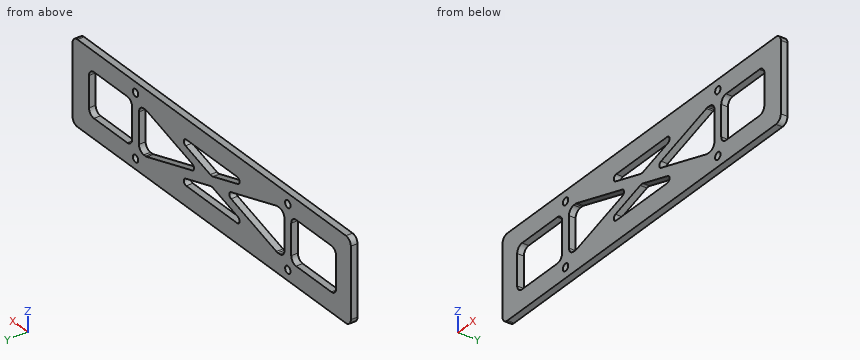
```python
from build123d import *

# Parameters (mm, degrees)
SKETCH1_W           = 145.0086
SKETCH1_H           = 32.004
SKETCH1_R           = 1.399999994
SKETCH1_R_2         = 1.399999995
SKETCH1_W_2         = 22.457386235
SKETCH1_H_2         = 16.9672
SKETCH1_W_3         = 23.43040653
BOSS_EXTRUDE1_DEPTH = 2.54
FILLET1_R           = 2.54
FILLET2_R           = 1.27


with BuildPart() as part:
    # Sketch1 → Boss-Extrude1 (new body)
    with BuildSketch(Plane(origin=(0, 0, 0), x_dir=(1, 0, 0), z_dir=(0, 1, 0))):
        with Locations((6.69779506, 14.755388179)):
            Rectangle(SKETCH1_W, SKETCH1_H)
        with Locations(Location((-32.97809841, 26.794988179, 0), (0, 0, 270))):
            Circle(SKETCH1_R, mode=Mode.SUBTRACT)
        with Locations(Location((46.373688528, 26.794988179, 0), (0, 0, 90))):
            Circle(SKETCH1_R_2, mode=Mode.SUBTRACT)
        with Locations(Location((46.373688528, 2.715788179, 0), (0, 0, 270))):
            Circle(SKETCH1_R_2, mode=Mode.SUBTRACT)
        with Locations(Location((-32.97809841, 2.715788179, 0), (0, 0, 90))):
            Circle(SKETCH1_R, mode=Mode.SUBTRACT)
        Polygon((-31.20009841, 23.238988179), (-27.382615546, 23.238988179), (0.574659599, 14.755388179), (-27.382615546, 6.271788179), (-31.20009841, 6.271788179), align=None, mode=Mode.SUBTRACT)
        with Locations((59.380381646, 14.755388179)):
            Rectangle(SKETCH1_W_2, SKETCH1_H_2, mode=Mode.SUBTRACT)
        with Locations((-46.471301675, 14.755388179)):
            Rectangle(SKETCH1_W_3, SKETCH1_H_2, mode=Mode.SUBTRACT)
        Polygon((40.778205663, 23.238988179), (12.820930519, 14.755388179), (40.778205663, 6.271788179), (44.595688528, 6.271788179), (44.595688528, 23.238988179), align=None, mode=Mode.SUBTRACT)
        Polygon((-15.136344626, 23.238988179), (6.697795059, 16.613445937), (28.531934744, 23.238988179), align=None, mode=Mode.SUBTRACT)
        Polygon((6.697795059, 12.897330421), (-15.136344626, 6.271788179), (28.531934744, 6.271788179), align=None, mode=Mode.SUBTRACT)
    extrude(amount=BOSS_EXTRUDE1_DEPTH)

    # Fillet1
    fillet1_edges = [part.edges().sort_by_distance(p)[0] for p in [
        (70.609074763, 1.27, -6.271788179),
        (70.609074763, 1.27, -23.238988179),
        (48.151688528, 1.27, -23.238988179),
        (48.151688528, 1.27, -6.271788179),
        (-58.18650494, 1.27, -23.238988179),
        (-58.18650494, 1.27, -6.271788179),
        (-34.75609841, 1.27, -6.271788179),
        (-34.75609841, 1.27, -23.238988179),
        (6.697795059, 1.27, -16.613445937),
        (6.697795059, 1.27, -12.897330421),
        (79.20209506, 1.27, 1.246611821),
        (-65.80650494, 1.27, 1.246611821),
        (-65.80650494, 1.27, -30.757388179),
        (79.20209506, 1.27, -30.757388179),
        (44.595688528, 1.27, -23.238988179),
        (40.778205663, 1.27, -23.238988179),
        (40.778205663, 1.27, -6.271788179),
        (44.595688528, 1.27, -6.271788179),
        (-31.20009841, 1.27, -23.238988179),
        (-31.20009841, 1.27, -6.271788179),
        (-27.382615546, 1.27, -6.271788179),
        (-27.382615546, 1.27, -23.238988179),
    ]]
    fillet(fillet1_edges, radius=FILLET1_R)

    # Fillet2
    fillet2_edges = [part.edges().sort_by_distance(p)[0] for p in [
        (28.531934744, 1.27, -23.238988179),
        (-15.136344626, 1.27, -23.238988179),
        (-15.136344626, 1.27, -6.271788179),
        (28.531934744, 1.27, -6.271788179),
        (12.820930519, 1.27, -14.755388179),
        (0.574659599, 1.27, -14.755388179),
    ]]
    fillet(fillet2_edges, radius=FILLET2_R)


solid = part.part
```
Geometry: final body of the model. Coordinates: model frame, mm. Coordinates: 2 decimals unless noted, no trailing zeros. Order: outer loops, then holes, each group sorted by start corner. A loop starts at its lowest first (then second) coordinate and runs counter-clockwise, first axis right, second up.
Item 1: Section query B-B (x = 4). Output: boundary loops of the cut face in (y, z), then the cut area to 3 significant figures.
Answer:
outline: (0, -30.76) - (2.54, -30.76) - (2.54, -23.24) - (0, -23.24) - close; (0, -17.43) - (2.54, -17.43) - (2.54, -12.08) - (0, -12.08) - close; (0, -6.27) - (2.54, -6.27) - (2.54, 1.25) - (0, 1.25) - close
area: 51.8 mm2
Item 2: Material intervals for line 1 along X through (y, z) = (2.25, -27); line 2 along Z through (x, y) = (-55, 0.9); line 3 along X through (y, z) = (1, -15), sorted ascending.
Answer:
line 1: x = -65.81 to -34.36, -31.59 to 44.99, 47.76 to 79.2
line 2: z = -30.76 to -23.24, -6.27 to 1.25
line 3: x = -65.81 to -58.19, -34.76 to -31.2, -2.55 to 15.95, 44.6 to 48.15, 70.61 to 79.2
Item 3: Section query C-C (x = -22). Output: boundary loops of the cut face in (y, z), then the cut area to 3 significant figures.
Answer:
outline: (0, -30.76) - (2.54, -30.76) - (2.54, -21.61) - (0, -21.61) - close; (0, -7.91) - (2.54, -7.91) - (2.54, 1.25) - (0, 1.25) - close
area: 46.5 mm2
Item 4: Section query D-D (y = 1.95). State how many separate pieces and enclosed holes the cut face has, then the cut area to 3 significant figures.
Answer:
separate pieces: 1
enclosed holes: 10
area: 3,000 mm2
Item 5: Section query A-A (x = 59). Output: boundary loops of the cut face in (y, z), then the cut area to 3 significant figures.
Answer:
outline: (0, -30.76) - (2.54, -30.76) - (2.54, -23.24) - (0, -23.24) - close; (0, -6.27) - (2.54, -6.27) - (2.54, 1.25) - (0, 1.25) - close
area: 38.2 mm2
